Read the model definition and answer for the solid it produces. Units are mm, in the model's axes. A direction names the side the tool comes from. Coordinates: 2 decimals unless noted, no trailing zeros. Order: outer loops, then holes, each group sorted by start corner. A loop starts at its lowest first (then second) coordinate and runs counter-clockwise, first axis right, second up. Notation, with made-up numbers: M -21,-39.75 L -6,-39.75 A14 cw -6,-12.75 Z; hole C 50,69 d1. An arc over 180 degrees is marked long. One line per question, with ' | ' between items. Start each with the question number.
1) Consider probe 1 along X at (y, z) = (0.5, 7.5) (3 decimals); probe 2 along Z at (x, y) = (61.5, -1.75); probe 3 along Y at (x, z) = (58, -0.5). Determine where each line is inside the solid, lowest interval first.
2) A tool of negligible diameter and unlimited length cuts with its end or side. For faces 1 (the face through (69.6, -2.09, -9.39)), 2 (the face through (-6.12, -0.69, -3.1)), from which of +Z, -Z, +X, -X, +Y, -Y can it reach the whole face along a straight path? Write none if from no direction.
3) Find section C-C, the plane x = 31. Write down the section's boundary in (y, z) (3 decimals), plus the area to 3 significant figures.
4) Given P1, Ø8, axis at x = 25.5, y = -6, coming from the +Z side; P2, Ø2, axis at x = 55.5, y = -2.5, coming from the +Z side; P3, Ø8, axis at y = -2, z = -6.5, coming from the -X side; P4, Ø1.5, axis at x = 47.5, z = 5.5, coming from the -Y side (3 decimals), each flat-ended and moving along its own axis, determine where each tip first touches the part or whether it passes through.
5) Find section A-A, the plane z = 0. Write down the section's boundary in (x, y) (3 decimals).
6) Find section D-D, the plane z = -8. Write down the section's boundary in (x, y) (3 decimals).
Autodesk Inventor part; units mm, degrees
ref_plane "dia1_XY" through (0, 3.175, 0) normal (1, 0, 0) x (0, 0, -1)
ref_plane "dia1_YZ" through (0, 3.175, 0) normal (0, 0, -1) x (0, 1, 0)
ref_plane "dia1_ZX" through (0, 3.175, 0) normal (0, 1, 0) x (1, 0, 0)
sketch "Sketch_1" plane through (0, 0, 0) normal (0, 0, 1) x (1, 0, 0)
  line L0 (79.375, 0) -> (0, 0)
  line L1 (0, 0) -> (0, 3.175)
  line L2 (0, 3.175) -> (59.5376, 3.175)
  line L3 (59.5376, 3.175) -> (59.5376, 9.6203)
  line L4 (59.5376, 9.6203) -> (79.375, 9.6203)
  line L5 (79.375, 9.6203) -> (79.375, 0)
  line L6 (79.375, 0) -> (0, 0)
revolve "Revolution1" add sketch "Sketch_1" angle 360 about axis through (79.375, 0, 0) along (1, 0, 0)
sketch "Sketch_3" plane through (0, 0, 0) normal (0, 0, 1) x (1, 0, 0)
  line L0 (0, 0) -> (-12.7, 0)
  line L1 (-12.7, 0) -> (-12.7, 2.634)
  line L2 (-12.7, 2.634) -> (-12.159, 3.175)
  line L3 (-12.159, 3.175) -> (0, 3.175)
  line L4 (0, 3.175) -> (0, 0)
  line L5 (0, 0) -> (-12.7, 0)
revolve "Revolution2" add sketch "Sketch_3" angle 360 about axis through (0, 0, 0) along (1, 0, 0)
thread "Thread1"
sketch "Sketch_30" plane through (0, 0, 0) normal (0, 0, 1) x (1, 0, 0)
  line L0 (0, 0) -> (-0.254, 0)
  line L1 (-0.254, 2.921) -> (0, 2.921)
  line L2 (0, 2.921) -> (0, 3.429)
  line L3 (0, 3.429) -> (-0.254, 3.429)
  line L4 (-0.254, 3.429) -> (-0.254, 2.921)
revolve "Revolution3" cut sketch "Sketch_30" angle 360 about axis through (0, 0, 0) along (1, 0, 0)
ref_plane "dia1_XY" through (0, 3.175, 0) normal (1, 0, 0) x (0, 0, -1)
ref_plane "dia1_YZ" through (0, 3.175, 0) normal (0, 0, -1) x (0, 1, 0)
ref_plane "dia1_ZX" through (0, 3.175, 0) normal (0, 1, 0) x (1, 0, 0)
ref_plane "dia12_XY" through (0, 0, 10.9537) normal (1, 0, 0) x (0, 0, -1)
ref_plane "dia12_YZ" through (0, 0, 10.9537) normal (0, 0, -1) x (0, 1, 0)
ref_plane "dia12_ZX" through (0, 0, 10.9537) normal (0, 1, 0) x (1, 0, 0)
ref_plane "dia1r_XY" through (0, 0, 10.2235) normal (1, 0, 0) x (0, 0, -1)
ref_plane "dia1r_YZ" through (0, 0, 10.2235) normal (0, 0, -1) x (0, 1, 0)
ref_plane "dia1r_ZX" through (0, 0, 10.2235) normal (0, 1, 0) x (1, 0, 0)
ref_plane "dia2_XY" through (0, -3.175, 0) normal (1, 0, 0) x (0, 0, -1)
ref_plane "dia2_YZ" through (0, -3.175, 0) normal (0, 0, -1) x (0, 1, 0)
ref_plane "dia2_ZX" through (0, -3.175, 0) normal (0, 1, 0) x (1, 0, 0)
ref_plane "dia22_XY" through (0, 0, -10.9537) normal (1, 0, 0) x (0, 0, -1)
ref_plane "dia22_YZ" through (0, 0, -10.9537) normal (0, 0, -1) x (0, 1, 0)
ref_plane "dia22_ZX" through (0, 0, -10.9537) normal (0, 1, 0) x (1, 0, 0)
ref_plane "dia2r_XY" through (0, 0, -10.2235) normal (1, 0, 0) x (0, 0, -1)
ref_plane "dia2r_YZ" through (0, 0, -10.2235) normal (0, 0, -1) x (0, 1, 0)
ref_plane "dia2r_ZX" through (0, 0, -10.2235) normal (0, 1, 0) x (1, 0, 0)
ref_plane "rl1_XY" through (-12.7, 0, 0) normal (1, 0, 0) x (0, 0, -1)
ref_plane "rl1_YZ" through (-12.7, 0, 0) normal (0, 0, -1) x (0, 1, 0)
ref_plane "rl1_ZX" through (-12.7, 0, 0) normal (0, 1, 0) x (1, 0, 0)
ref_plane "rl2_XY" through (0, 0, 0) normal (1, 0, 0) x (0, 0, -1)
ref_plane "rl2_YZ" through (0, 0, 0) normal (0, 0, -1) x (0, 1, 0)
ref_plane "rl2_ZX" through (0, 0, 0) normal (0, 1, 0) x (1, 0, 0)
ref_plane "rod_cp_XY" through (0, 0, 0) normal (1, 0, 0) x (0, 0, -1)
ref_plane "rod_cp_YZ" through (0, 0, 0) normal (0, 0, -1) x (0, 1, 0)
ref_plane "rod_cp_ZX" through (0, 0, 0) normal (0, 1, 0) x (1, 0, 0)
ref_plane "stroke1_XY" through (0, 0, 0) normal (1, 0, 0) x (0, 0, -1)
ref_plane "stroke1_YZ" through (0, 0, 0) normal (0, 0, -1) x (0, 1, 0)
ref_plane "stroke1_ZX" through (0, 0, 0) normal (0, 1, 0) x (1, 0, 0)
ref_plane "thd1_XY" through (-12.7, 3.175, 0) normal (1, 0, 0) x (0, 0, -1)
ref_plane "thd1_YZ" through (-12.7, 3.175, 0) normal (0, 0, -1) x (0, 1, 0)
ref_plane "thd1_ZX" through (-12.7, 3.175, 0) normal (0, 1, 0) x (1, 0, 0)
ref_plane "thd2_XY" through (-12.7, -3.175, 0) normal (1, 0, 0) x (0, 0, -1)
ref_plane "thd2_YZ" through (-12.7, -3.175, 0) normal (0, 0, -1) x (0, 1, 0)
ref_plane "thd2_ZX" through (-12.7, -3.175, 0) normal (0, 1, 0) x (1, 0, 0)
ref_plane "to_rod_clevis_XY" through (-16.764, 0, 0) normal (1, 0, 0) x (0, 0, -1)
ref_plane "to_rod_clevis_YZ" through (-16.764, 0, 0) normal (0, 0, -1) x (0, 1, 0)
ref_plane "to_rod_clevis_ZX" through (-16.764, 0, 0) normal (0, 1, 0) x (1, 0, 0)
properties part number "C-040.75-R0000_rod"
Report:
1) probe 1: x = 59.538 to 79.375 | probe 2: z = -9.46 to 9.46 | probe 3: y = -3.14 to 3.14
2) face 1: +X, -X | face 2: -X
3) outline: C 0,0 d6.35 | area: 31.7 mm^2
4) P1: stops at z = 2.47 | P2: stops at z = 2.8 | P3: stops at x = -12.53 | P4: passes through
5) outline: M -12.7,-2.634 L -12.159,-3.175 L -0.254,-3.175 L -0.254,-2.921 L 0,-2.921 L 0,-3.175 L 59.538,-3.175 L 59.538,-9.62 L 79.375,-9.62 L 79.375,9.62 L 59.538,9.62 L 59.538,3.175 L 0,3.175 L 0,2.921 L -0.254,2.921 L -0.254,3.175 L -12.159,3.175 L -12.7,2.634 Z
6) outline: M 59.538,-5.343 L 79.375,-5.343 L 79.375,5.343 L 59.538,5.343 Z
